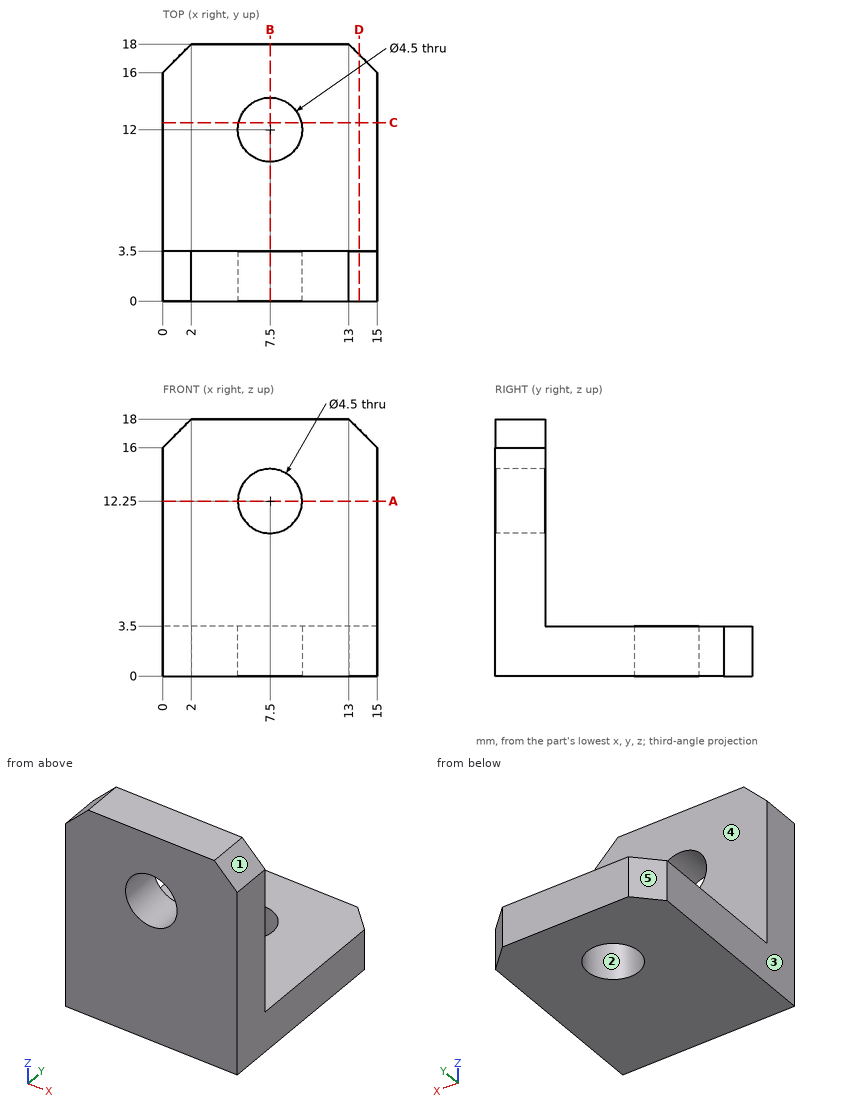
The figure shows three views and two pictorial views of one solid part (mm, origin at its lowest corner). Answer the questions. A direction names the side the tool comes from. Round coordinates to 2 decimals unless told otherwise and drop trailing zeros. Loops run counter-clockwise (first coordinate to the right, second up) from the corner with the lowest first, then second, coordinate; pieces in that order, holes last. Notation, with made-up numbers: (3.25, -33) - (20.25, -33) arc R33 ccw to (20.25, 5) - close; hole circle Ø3 at (66, 51). An arc over 180 degrees is marked (long way). One line per question, with ' | ' between items. Start each with the question number.
Q1. Find the intervals of material crossed by L1, parallel to Z at x = 7.5, y = 2.25; L2, parallel to Y at x = 7.5, z = 1.55; L3, parallel to Z at x = 13.25, y = 8.25, in increasing order.
Q2. For a pull along X with two mould halves and no side action, classify the marked faces 1, 2 and 3 as +X half, -X half, draft (parallel to the pull), parting line (faces both ways), or undercut.
Q3. Flat-ended cylindrical pins translate along their axes: pin 1 (7 mm diameter, centred on x = 7.5, y = 12, fed in from -Z); pin 2 (1 mm diameter, centred on x = 2.5, y = 10, fed in from +Z); pin 3 (6 mm diameter, centred on x = 12.5, z = 8, fed in from +Y). Find the tip coordinate at first contact, or state that the pin passes through.
Q4. Section A-A on z = 12.25 is taken. Give the vertices of the cut face in (x, y).
Q5. Section D-D on x = 13.75 is taken. Give the vertices of the cut face in (y, z).
Q6. For the marked faces 4 and 5, determine the directions among +Z, -Z, +X, -X, +Y, -Y from which every point of the face is accessible in a straight line to the end or side of a thin tool.
Q7. Section B-B on x = 7.5 is taken. Give the vertices of the cut face in (y, z).
Q8. Section C-C on y = 12.5 is taken. Give the vertices of the cut face in (x, z), plus the area to 3 significant figures.
Established:
1) L1: 0 to 10, 14.5 to 18 | L2: 0 to 9.75, 14.25 to 18 | L3: 0 to 3.5
2) face 1: +X half | face 2: undercut | face 3: -X half
3) pin 1: z = 0 | pin 2: z = 3.5 | pin 3: y = 3.5
4) outline: (0, 0) - (5.25, 0) - (5.25, 3.5) - (0, 3.5) - close; (9.75, 0) - (15, 0) - (15, 3.5) - (9.75, 3.5) - close
5) outline: (0, 0) - (17.25, 0) - (17.25, 3.5) - (3.5, 3.5) - (3.5, 17.25) - (0, 17.25) - close
6) face 4: +Z, +X, -X, +Y | face 5: +Z, -Z, -X, +Y
7) outline: (0, 0) - (9.75, 0) - (9.75, 3.5) - (3.5, 3.5) - (3.5, 10) - (0, 10) - close; (0, 14.5) - (3.5, 14.5) - (3.5, 18) - (0, 18) - close; (14.25, 0) - (18, 0) - (18, 3.5) - (14.25, 3.5) - close
8) outline: (0, 0) - (5.31, 0) - (5.31, 3.5) - (0, 3.5) - close; (9.69, 0) - (15, 0) - (15, 3.5) - (9.69, 3.5) - close | area: 37.1 mm²
